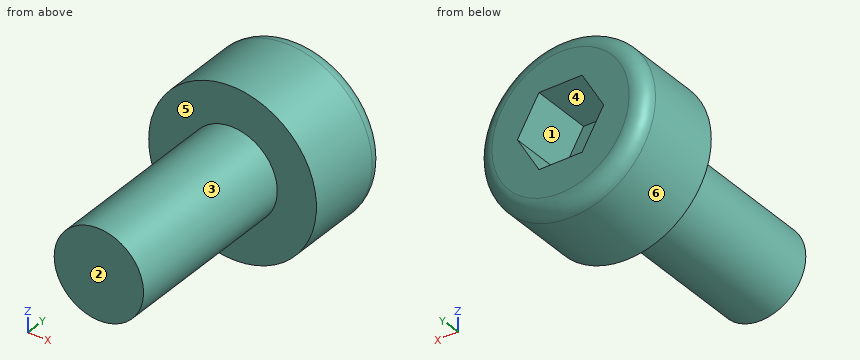
Autodesk Inventor part; units mm, degrees
ref_plane "YZ Plane" through (0, 0, 0) normal (1, 0, 0) x (0, 1, 0)
ref_plane "XZ Plane" through (0, 0, 0) normal (0, 1, 0) x (-1, 0, 0)
ref_plane "XY Plane" through (0, 0, 0) normal (0, 0, 1) x (1, 0, 0)
sketch "Sketch1" plane through (0, 0, 0) normal (0, 1, 0) x (-1, 0, 0)
  circle A0 centre (0, 0) radius 1.465
  circle A1 centre (0, 0) radius 2.75
  line L0 (0.7073, -1.225) -> (-0.7073, -1.225)
  line L1 (-0.7073, -1.225) -> (-1.4145, 0)
  line L2 (-1.4145, 0) -> (-0.7073, 1.225)
  line L3 (-0.7073, 1.225) -> (0.7073, 1.225)
  line L4 (0.7073, 1.225) -> (1.4145, 0)
  line L5 (1.4145, 0) -> (0.7073, -1.225)
  dimension "d0" = 2.93
  dimension "d1" = 5.5
  dimension "d8" = 2.45
extrude "Extrusion1" add sketch "Sketch1" along normal blind 3 contours A0 | A1 | L0 L1 L2 L3 L4 L5
extrude "Extrusion2" add sketch "Sketch1" against normal blind 6 contours A0 | L0 L1 L2 L3 L4 L5
extrude "Extrusion3" cut sketch "Sketch1" against normal blind 2 from surface at 3 contours L0 L1 L2 L3 L4 L5
fillet "Fillet1" radius 0.5 1 edges at (2.75, 3, 0)
thread "Thread2"
equation "\"d4\" = length"
equation "\"length\" = 6"
properties part number "M3x16"
CAD build for the part. Positions are in the model's coordinates, mm. Face numbers are marked on the shaded views. A direction names the side the tool comes from. Give positions to 0.01 mm unless a question says otherwise; leave off trailing zeros. Write each loop counter-clockwise with the first axis right and the second up, starting at its lowest first coordinate (ties: lowest second). Pieces come first, ordered by that corner, then holes. Notation, with made-up numbers: M -15,77 L 23,77 A19 cw 23,92 Z; hole C 67,52 d2. An arc over 180 degrees is marked long. Return JSON: item names as keys, results as strings. Group by question number.
(1) Mould opens along Z. For the marked faces 1, 2 and 3 say: pulls with the +Z half, pulls with the -Z half, needs draft (parallel to the pull), parting line crosses it, or undercut.
(2) 3-axis set-ups, long thin cutter, end or side, ignore diameter. For the marked faces 4, 5 and 6: which of +Z, -Z, +X, -X, +Y, -Y reach the whole face in a straight line?
(3) Drill centre lines: L1, parallel to Y at x = -1, z = 1.45; L2, parallel to Y at x = -0.1, z = -0.1; L3, parallel to Z at x = 1, y = -3. Where is each one in solid material? Low to high. Write a range as [from, to].
(4) Band-saw the part on C-C (y = -2.25). Give the cut face in (x, z) (3 decimals).
(5) Band-saw the part on B-B (x = 0). Give the cut face in (y, z) (3 decimals), and give its area (3 significant figures).
(6) Flat gauge pins, fed straight in: pin 1 Ø2 at (x, z) = (0.5, -0.5) entering from +Y; pin 2 Ø1.5 at (y, z) = (-2.5, 0) entering from -X (3 decimals); pin 3 Ø1 at (x, y) = (2, -4.5) entering from -Z; pin 4 Ø0.7 at (x, y) = (-0.5, 2) entering from +Z. Where does each tip first touch, or does it go through?
Entries:
{
 "1": {"face 1": "undercut", "face 2": "needs draft", "face 3": "parting line crosses it"},
 "2": {"face 4": "+Y", "face 5": "-Y", "face 6": "+Y, -Y"},
 "3": {"L1": "y = [0, 3]", "L2": "y = [-6, 1]", "L3": "z = [-1.07, 1.07]"},
 "4": {"outline": "C 0,0 d2.93"},
 "5": {"outline": "M -6,-1.465 L 0,-1.465 L 0,-2.75 L 2.5,-2.75 A0.5 ccw 3,-2.25 L 3,-1.225 L 1,-1.225 L 1,1.225 L 3,1.225 L 3,2.25 A0.5 ccw 2.5,2.75 L 0,2.75 L 0,1.465 L -6,1.465 Z", "area": "29.1 mm^2"},
 "6": {"pin 1": "stops at y = 3", "pin 2": "stops at x = -1.465", "pin 3": "passes through", "pin 4": "stops at z = 2.75"}
}
